Input: dimensioned drawing with shaded views. Units: mm. Origin: part minimum x, y, z. Round coordinates to 2 decimals unless told otherwise and drop trailing zeros. Order: outer loops, then holes, each group sorted by start corner. A loop starts at its lowest first (then second) coordinate and runs counter-clockwise, first axis right, second up. Notation, with made-up numbers: (-2.75, 33.25) - (3.25, 33.25) arc R33 cw to (3.25, 61.25) - close; hole circle Ø9 at (10.5, -1.75). An arc over 180 degrees is marked (long way). Put each result on its own line as item: value. Start each with the question number.
(1) Section A-A (x = 2). Count the separate pieces of the cut face and the enclosed holes in it, and give its area (3 significant figures).
(2) Section B-B (y = 33.02). Output: boundary loops of the cut face in (x, z).
(3) Material intervals for L1, parallel to Y at x = 2, z = 19.05; L2, parallel to Y at x = 0.55, z = 26 (1 decimal); L3, parallel to Z at x = 0.85, y = 43.5, sorted ascending. Write a range as [from, to].
(4) Section D-D (y = 6). Output: boundary loops of the cut face in (x, z), and give its area (3 significant figures).
(5) Section C-C (z = 19.05). Output: boundary loops of the cut face in (x, y).
(6) Pin query (flat end, axial travel): P1, Ø1.3, axis at x = 1, y = 36, coming from the +Z side; P2, Ø0.8, axis at x = 2, z = 2, coming from the -Y side (3 decimals); P3, Ø0.8, axis at x = 1, y = 7.5, coming from the -Z side; P4, Ø4.5, axis at y = 33.02, z = 19.05, coming from the +X side. Return the tip coordinate at first contact, or that it passes through.
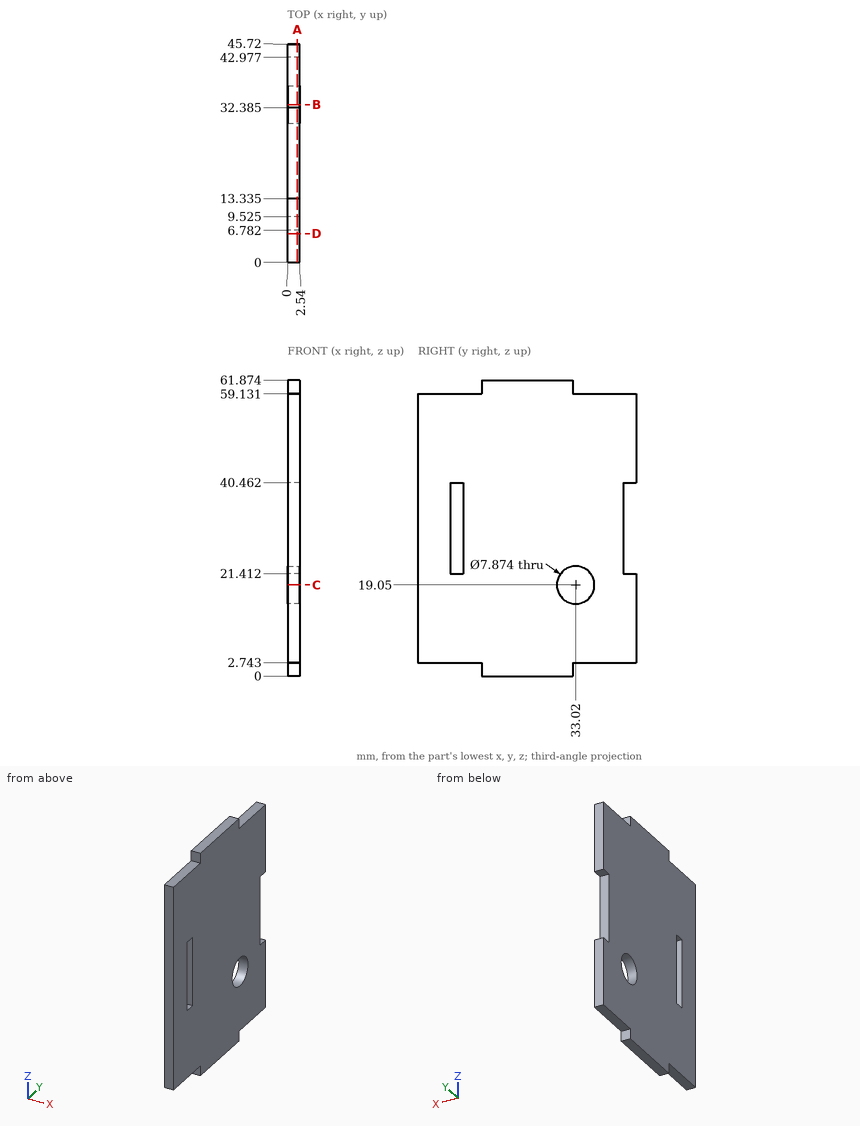
Checks:
1. separate pieces: 1
1. enclosed holes: 2
1. area: 2,530 mm²
2. outline: (0, 2.74) - (2.54, 2.74) - (2.54, 15.11) - (0, 15.11) - close; (0, 22.99) - (2.54, 22.99) - (2.54, 59.13) - (0, 59.13) - close
3. L1: y = [0, 29.08], [36.96, 45.72]
3. L2: y = [0, 6.8], [9.5, 43]
3. L3: z = [2.74, 21.41], [40.46, 59.13]
4. outline: (0, 2.74) - (2.54, 2.74) - (2.54, 59.13) - (0, 59.13) - close
4. area: 143 mm²
5. outline: (0, 0) - (2.54, 0) - (2.54, 29.08) - (0, 29.08) - close; (0, 36.96) - (2.54, 36.96) - (2.54, 45.72) - (0, 45.72) - close
6. P1: stops at z = 59.13
6. P2: stops at y = 13.335
6. P3: stops at z = 2.74
6. P4: passes through
